Check sheet for the drawn part. Datum: minimum x, y, z corner. Units: mm. Give positions to 0.01 mm unless a question says otherwise; leave off trailing zeros. Write each loop counter-clockwise with the first axis right and the second up, starting at its lowest first coordinate (ties: lowest second). Pieces come first, ordered by that corner, then holes. Notation, with made-up numbers: M -29,12.5 L 17,12.5 A26 ccw 17,36.5 Z; hole C -30.5,69 d1. An arc over 180 degrees is marked long. Use CSV: the item, a comma, the result in double quotes. Start each with the question number.
1. Cross-section at C-C, the plane y = 67. Enter the section's corners in (x, z) (1 decimal).
2. Cross-section at B-B, the plane x = 11. Enter the section's corners in (y, z).
3. Depth check by flat-ended pin: P1, Ø5, axis at x = 8.94, y = 9.98, coming from the +Z side. Enter the tip coordinate at first touch or a pass-through.
4. Cross-section at A-A, the plane z = 1.25. Enter the section's corners in (x, y) (1 decimal), and give its area (3 significant figures).
5. Scan lines: line 1 (X direction, y = 75, z = 0.4) (1 decimal); line 2 (X direction, y = 72.5, z = 0.35) (1 decimal); line 3 (Y direction, x = 62, z = 2.25). Record each from-to range of solid material in increasing order.
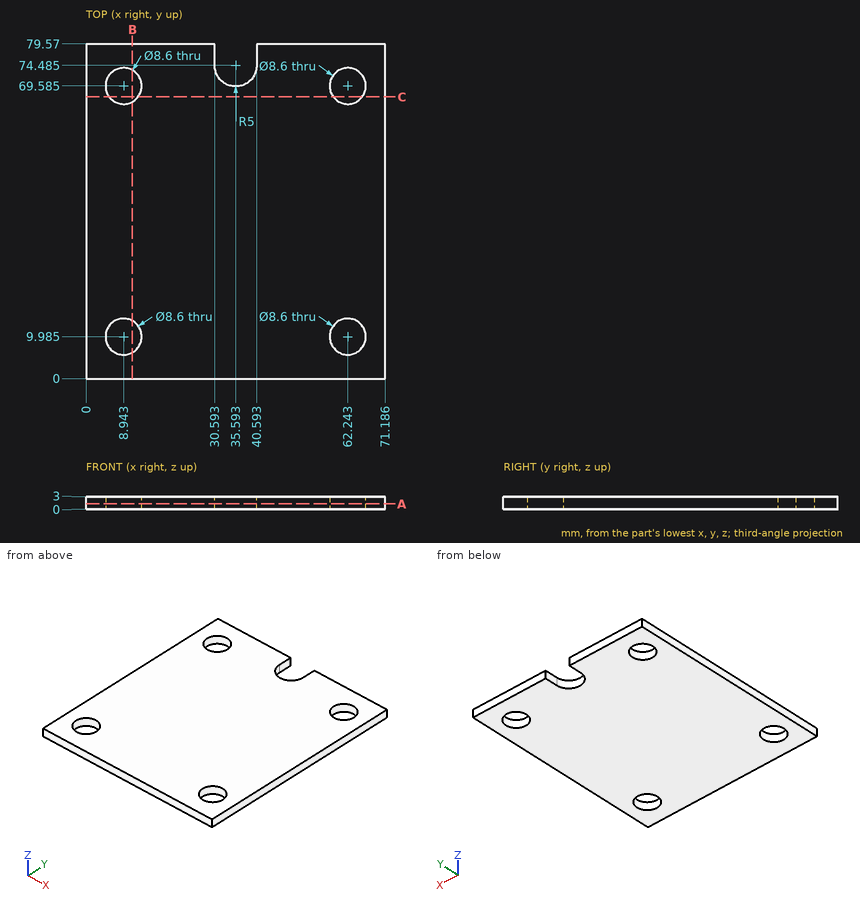
Worked answers:
1,outline,"M 0,0 L 5.5,0 L 5.5,3 L 0,3 Z; M 12.4,0 L 58.8,0 L 58.8,3 L 12.4,3 Z; M 65.7,0 L 71.2,0 L 71.2,3 L 65.7,3 Z"
2,outline,"M 0,0 L 6.21,0 L 6.21,3 L 0,3 Z; M 13.76,0 L 65.81,0 L 65.81,3 L 13.76,3 Z; M 73.36,0 L 79.57,0 L 79.57,3 L 73.36,3 Z"
3,P1,"passes through"
4,outline,"M 0,0 L 71.2,0 L 71.2,79.6 L 40.6,79.6 L 40.6,74.5 A5 cw 30.6,74.5 L 30.6,79.6 L 0,79.6 Z; hole C 8.9,10 d8.6; hole C 8.9,69.6 d8.6; hole C 62.2,10 d8.6; hole C 62.2,69.6 d8.6"
4,area,"5,340 mm^2"
5,line 1,"x = 0 to 30.6, 40.6 to 71.2"
5,line 2,"x = 0 to 5.8, 12.1 to 31, 40.2 to 59.1, 65.4 to 71.2"
5,line 3,"y = 0 to 5.69, 14.28 to 65.29, 73.88 to 79.57"
